Work out the finished part from the listing and answer in its coordinate system (mm). A direction names the side the tool comes from. Round coordinates to 2 decimals unless told otherwise and drop trailing zeros. Write each loop counter-clockwise with the first axis right and the second up, starting at its lowest first coordinate (ties: lowest second). Pieces come first, ordered by that corner, then holes.
from build123d import *

# Parameters (mm, degrees)
SKETCH1_W               = 90
SKETCH1_H               = 12
BOSS_EXTRUDE1_DEPTH     = 2
SKETCH2_W               = 90
SKETCH2_H               = 2
BOSS_EXTRUDE2_DEPTH     = 10
CUT_EXTRUDE1_DEPTH      = 63.420894383
CUT_EXTRUDE1_DEPTH_BACK = 63.420894383
SKETCH3_R               = 2.5


with BuildPart() as part:
    # Sketch1 → Boss-Extrude1 (new body)
    with BuildSketch(Plane(origin=(0, 0, 0), x_dir=(1, 0, 0), z_dir=(0, 1, 0))):
        with Locations((-16.166666667, 1.416666667)):
            Rectangle(SKETCH1_W, SKETCH1_H)
    extrude(amount=BOSS_EXTRUDE1_DEPTH)

    # Sketch2 → Boss-Extrude2 (add)
    with BuildSketch(Plane(origin=(0, 2, 0), x_dir=(1, 0, 0), z_dir=(0, 1, 0))):
        with Locations((-16.166666667, 6.416666667)):
            Rectangle(SKETCH2_W, SKETCH2_H)
    extrude(amount=BOSS_EXTRUDE2_DEPTH)

    # Sketch3 → Cut-Extrude1 (cut, two sides: drawn at the far end of the back side and taken through both)
    with BuildSketch(Plane(origin=(0, 2, 0), x_dir=(1, 0, 0), z_dir=(0, 1, 0)).offset(-CUT_EXTRUDE1_DEPTH_BACK)):
        with Locations(Location((-28.666666667, 0, 0), (0, 0, 270))):
            Circle(SKETCH3_R)
        with Locations(Location((-3.666666667, 0, 0), (0, 0, 270))):
            Circle(SKETCH3_R)
    extrude(amount=CUT_EXTRUDE1_DEPTH + CUT_EXTRUDE1_DEPTH_BACK, mode=Mode.SUBTRACT)


solid = part.part
Q1. A tool of negligible diameter and unlimited length cuts with its end or side. For faces 1 (the face through (-17, 2, 0)), 2 (the face through (-17, 12, -6)), from which of +Z, -Z, +X, -X, +Y, -Y can it reach the whole face along a straight path? Write none if from no direction.
Q2. Find section D-D (y = 4.5). Determine the outline of the cut face in (x, z), plus the area to 3 significant figures.
Q3. Given pin 1 (5 mm diameter, centred on x = -0.5, y = 7.5, fed in from +Z), flat-ended and moving along its own axis, determine where the tip first touches the part or whether it passes through.
Q4. The mould has two halves that part along X. Classify faces 3 (the face through (-17, 1, 4.583)), 4 (the face through (-61.167, 1, -3)), 5 (the face through (28.833, 1, -3)), 6 (the face through (-2.916, 0.986, 2.385)): +X half, -X half, draft (parallel to the pull), parting line (faces both ways), or undercut.
Q5. Find section A-A (z = 0). Determine the outline of the cut face in (x, y), plus the area to 3 significant figures.
Q6. Find section B-B (x = 0). Determine the outline of the cut face in (y, z).
Q7. Find section C-C (z = -3.75). Determine the outline of the cut face in (x, y).
Q8. Find the intervals of material crossed by L1, parallel to X at y = 0.55, z = 0; L2, parallel to X at y = 0.5, z = -2.25; L3, parallel to Z at x = 14, y = 3.75, in increasing order.
Report:
1. face 1: +Z, +X, -X, +Y
1. face 2: +Z, -Z, +X, -X, +Y
2. outline: (-61.17, -7.42) - (28.83, -7.42) - (28.83, -5.42) - (-61.17, -5.42) - close
2. area: 180 mm2
3. pin 1: stops at z = -5.42
4. face 3: draft
4. face 4: -X half
4. face 5: +X half
4. face 6: undercut
5. outline: (-61.17, 0) - (-31.17, 0) - (-31.17, 2) - (-61.17, 2) - close; (-26.17, 0) - (-6.17, 0) - (-6.17, 2) - (-26.17, 2) - close; (-1.17, 0) - (28.83, 0) - (28.83, 2) - (-1.17, 2) - close
5. area: 160 mm2
6. outline: (0, -7.42) - (12, -7.42) - (12, -5.42) - (2, -5.42) - (2, 4.58) - (0, 4.58) - close
7. outline: (-61.17, 0) - (28.83, 0) - (28.83, 2) - (-61.17, 2) - close
8. L1: x = -61.17 to -31.17, -26.17 to -6.17, -1.17 to 28.83
8. L2: x = -61.17 to -29.76, -27.58 to -4.76, -2.58 to 28.83
8. L3: z = -7.42 to -5.42
